Read the model definition and answer for the solid it produces. Units are mm, in the model's axes. A direction names the side the tool comes from. Give positions to 0.01 mm unless a question says otherwise; leave off trailing zeros. Order: outer loops, then holes, each group sorted by start corner. A loop starts at its lowest first (then second) coordinate and runs counter-clockwise, first axis right, second up. Notation, with made-up numbers: (-37.75, 83.25) - (-25.75, 83.25) arc R19 cw to (-25.75, 114.25) - close; hole circle Ø5 at (51, -1). An arc over 180 degrees is marked (long way). Write item = value, one per line.
```python
from build123d import *

# Parameters (mm, degrees)
BOSS_EXTRUDE1_DEPTH = 3


with BuildPart() as part:
    # Sketch1 → Boss-Extrude1 (new body)
    with BuildSketch(Plane.XY):
        Polygon((237, 253.5), (241.5, 253.5), (241.5, 262.5), (237, 262.5), (237, 265.5), (241.5, 265.5), (241.5, 274.5), (232.5, 274.5), (232.5, 270), (229.5, 270), (229.5, 274.5), (220.5, 274.5), (220.5, 270), (217.5, 270), (217.5, 274.5), (208.5, 274.5), (208.5, 270), (205.5, 270), (205.5, 274.5), (196.5, 274.5), (196.5, 270), (193.5, 270), (193.5, 274.5), (184.5, 274.5), (184.5, 270), (181.5, 270), (181.5, 274.5), (172.5, 274.5), (172.5, 270), (169.5, 270), (169.5, 274.5), (160.5, 274.5), (160.5, 265.5), (165, 265.5), (165, 262.5), (160.5, 262.5), (160.5, 253.5), (165, 253.5), (165, 250.5), (160.5, 250.5), (160.5, 241.5), (165, 241.5), (165, 238.5), (160.5, 238.5), (160.5, 229.5), (165, 229.5), (165, 226.5), (160.5, 226.5), (160.5, 217.5), (165, 217.5), (165, 214.5), (160.5, 214.5), (160.5, 205.5), (165, 205.5), (165, 202.5), (160.5, 202.5), (160.5, 193.5), (169.5, 193.5), (169.5, 198), (172.5, 198), (172.5, 193.5), (181.5, 193.5), (181.5, 198), (184.5, 198), (184.5, 193.5), (193.5, 193.5), (193.5, 198), (196.5, 198), (196.5, 193.5), (205.5, 193.5), (205.5, 198), (208.5, 198), (208.5, 193.5), (217.5, 193.5), (217.5, 198), (220.5, 198), (220.5, 193.5), (229.5, 193.5), (229.5, 198), (232.5, 198), (232.5, 193.5), (241.5, 193.5), (241.5, 202.5), (237, 202.5), (237, 205.5), (241.5, 205.5), (241.5, 214.5), (237, 214.5), (237, 217.5), (241.5, 217.5), (241.5, 226.5), (237, 226.5), (237, 229.5), (241.5, 229.5), (241.5, 238.5), (237, 238.5), (237, 241.5), (241.5, 241.5), (241.5, 250.5), (237, 250.5), align=None)
        with BuildLine():
            Line((180, 204), (171, 213))
            ThreePointArc((171, 213), (177.431527234, 234), (171, 255))
            Line((171, 255), (180, 264))
            ThreePointArc((180, 264), (201, 257.568472766), (222, 264))
            Line((222, 264), (231, 255))
            ThreePointArc((231, 255), (224.568472766, 234), (231, 213))
            Line((231, 213), (222, 204))
            ThreePointArc((222, 204), (201, 210.431527234), (180, 204))
        make_face(mode=Mode.SUBTRACT)
    extrude(amount=BOSS_EXTRUDE1_DEPTH)


solid = part.part
```
1. Section A-A (x = 209.5) is taken. Determine the outline of the cut face in (y, z), and give its area (3 significant figures).
Recorded:
outline = (193.5, 0) - (209.46, 0) - (209.46, 3) - (193.5, 3) - close; (258.54, 0) - (274.5, 0) - (274.5, 3) - (258.54, 3) - close
area = 95.7 mm^2
2. Flat-ended cylindrical pins translate along their axes: pin 1 (0.9 mm diameter, centred on x = 183.5, z = 1, fed in from -Y); pin 2 (1.5 mm diameter, centred on y = 228.5, z = 1, fed in from -X). Find the tip coordinate at first contact, or state that the pin passes through.
Recorded:
pin_1 = 198
pin_2 = 165
3. Determine the mould class of faces 4 (the face through (171, 270, 1)), 5 (the face through (163, 217.5, 1)), 6 (the face through (241.5, 222, 1)) for opening direction X: +X half, -X half, draft (parallel to the pull), parting line (faces both ways), or undercut.
Recorded:
face_4 = undercut
face_5 = draft
face_6 = +X half
4. Section B-B (y = 230.5) is taken. Determine the outline of the cut face in (x, z).
Recorded:
outline = (160.5, 0) - (177.27, 0) - (177.27, 3) - (160.5, 3) - close; (224.73, 0) - (241.5, 0) - (241.5, 3) - (224.73, 3) - close
5. Section C-C (y = 260) is taken. Determine the outline of the cut face in (x, z), and give its area (3 significant figures).
Recorded:
outline = (160.5, 0) - (176, 0) - (176, 3) - (160.5, 3) - close; (187.72, 0) - (214.28, 0) - (214.28, 3) - (187.72, 3) - close; (226, 0) - (241.5, 0) - (241.5, 3) - (226, 3) - close
area = 173 mm^2
6. Straight lines are drawn through the part: L1, parallel to X at y = 262, z = 0.4; L2, parallel to Y at x = 231.5, z = 0.5; L3, parallel to Y at x = 201.5, z = 1.7. For each, find the intervals that lie inside material, in ascending order. Write a range as [from, to].
Recorded:
L1 = [160.5, 178], [183.32, 218.68], [224, 241.5]
L2 = [198, 270]
L3 = [193.5, 210.43], [257.57, 274.5]
7. For faces 1 (the face through (231, 198, 1)), 2 (the face through (227, 209, 1)), 3 (the face through (239, 214.5, 1)), determine the directions among +Z, -Z, +X, -X, +Y, -Y from which every point of the face is accessible in a straight line to the end or side of a thin tool.
Recorded:
face_1 = +Z, -Z, -Y
face_2 = +Z, -Z
face_3 = +Z, -Z, +X
